from build123d import *

# Parameters (mm, degrees)
F0_W     = 20
F0_H     = 55
F1_DEPTH = 25.5
F3_DEPTH = 16
F5_DEPTH = 25
F7_D     = 5
F7_DEPTH = 10
F7_TIP   = 1.5021515476
F9_D     = 8
F9_DEPTH = 10
F9_TIP   = 2.4034424761


with BuildPart() as f1:
    # F0 (on Top) → F1 (new body)
    with BuildSketch(Plane.XY):
        Rectangle(F0_W, F0_H)
    extrude(amount=F1_DEPTH)

    # F2 (on face) → F3 (cut)
    with BuildSketch(Plane.XY.offset(25.5)):
        with BuildLine():
            Line((5, 10), (-5, 10))
            ThreePointArc((-5, 10), (-5.7071067812, 9.7071067812), (-6, 9))
            Line((-6, 9), (-6, -9))
            ThreePointArc((-6, -9), (-5.7071067812, -9.7071067812), (-5, -10))
            Line((-5, -10), (5, -10))
            ThreePointArc((5, -10), (5.7071067812, -9.7071067812), (6, -9))
            Line((6, -9), (6, 9))
            ThreePointArc((6, 9), (5.7071067812, 9.7071067812), (5, 10))
        make_face()
    extrude(amount=-F3_DEPTH, mode=Mode.SUBTRACT)

    # F4 (on face) → F5 (cut)
    with BuildSketch(Plane.YZ.offset(10)):
        Polygon((-27.5, 0), (-18, 0), (-15, 5.5), (-27.5, 5.5), align=None)
        Polygon((27.5, 5.5), (15, 5.5), (18, 0), (27.5, 0), align=None)
    extrude(amount=-F5_DEPTH, mode=Mode.SUBTRACT)

    # F7
    with Locations(Plane.YZ.offset(10)):
        with Locations((-17.5, 16.5), (17.5, 16.5)):
            Hole(F7_D / 2, depth=F7_DEPTH)
            with Locations((0, 0, -(F7_DEPTH + F7_TIP / 2))):  # 118° drill point
                Cone(0, F7_D / 2, F7_TIP, mode=Mode.SUBTRACT)

    # F9
    with Locations(Plane(origin=(-10, 0, 0), x_dir=(0, -1, 0), z_dir=(-1, 0, 0))):
        with Locations((0, 16.5)):
            Hole(F9_D / 2, depth=F9_DEPTH)
            with Locations((0, 0, -(F9_DEPTH + F9_TIP / 2))):  # 118° drill point
                Cone(0, F9_D / 2, F9_TIP, mode=Mode.SUBTRACT)


solid = f1.part
Here's how the part is built. I have some questions about the finished solid (model axes, mm). A direction names the side the tool comes from. Coordinates: 2 decimals unless noted, no trailing zeros. Order: outer loops, then holes, each group sorted by start corner. A loop starts at its lowest first (then second) coordinate and runs counter-clockwise, first axis right, second up. Notation, with made-up numbers: (-39, -24.5) - (3, -24.5) arc R25 ccw to (3, -1.5) - close; hole circle Ø2 at (18, 37.25). An arc over 180 degrees is marked (long way). Use CSV: the item, a comma, the result in double quotes. Start each with the question number.
1. Please list where these lines run through material, in increasing order: line 1 (X direction, y = 7.5, z = 22.5); line 2 (Y direction, x = 4.5, z = 20); line 3 (Y direction, x = 6.5, z = 16.5). Write a range as from..to.
2. Suppose I cut it at A-A on x = -8. List the corners of the cut face in (y, z) for me.
3. Suppose I cut it at C-C on x = -3.5. List the corners of the cut face in (y, z) for me.
4. If we mould it in two halves opening along Z, with no side actions, what happens to faces 4 (the face through (0, 0, 0)), 5 (the face through (-5.699, 9.715, 17.612)), 6 (the face through (4.9, -15, 16.6)), 7 (the face through (0.14, 16.48, 2.79))? For each: +Z half, -Z half, draft (parallel to the pull), parting line (faces both ways), or undercut.
5. Suppose I cut it at B-B on y = 0. List the corners of the cut face in (x, z) for me, then the cut area to 3 significant figures.
6. I'm going to push flat-ended pins straight in: pin 1 (10 mm diameter, centred on x = -2, y = 23.5, fed in from -Z); pin 2 (8 mm diameter, centred on y = -17.5, z = 16.5, fed in from +X); pin 3 (6 mm diameter, centred on x = -0.5, y = 5, fed in from +Z); pin 4 (1.5 mm diameter, centred on y = 0, z = 15, fed in from -X). Where does each tip first touch, or does it pass through?
7. Suppose I cut it at D-D on y = -6. List the corners of the cut face in (x, z) for me.
8. For faces 1 (the face through (6, 0, 18)), 2 (the face through (0.14, -16.52, 2.71)), 3 (the face through (4.9, 20, 16.6)), which set-ups out of +Z, -Z, +X, -X, +Y, -Y let a thin tool reach every point of the face, with its end or its side?
Output:
1,line 1,"x = -10..-6, 6..10"
1,line 2,"y = -27.5..-10, 10..27.5"
1,line 3,"y = -27.5..-20, -15..15, 20..27.5"
2,outline,"(-27.5, 5.5) - (-15, 5.5) - (-18, 0) - (18, 0) - (15, 5.5) - (27.5, 5.5) - (27.5, 25.5) - (-27.5, 25.5) - close; hole circle Ø8 at (0, 16.5)"
3,outline,"(-27.5, 5.5) - (-15, 5.5) - (-18, 0) - (18, 0) - (15, 5.5) - (27.5, 5.5) - (27.5, 25.5) - (10, 25.5) - (10, 9.5) - (-10, 9.5) - (-10, 25.5) - (-27.5, 25.5) - close"
4,face 4,"-Z half"
4,face 5,"draft"
4,face 6,"undercut"
4,face 7,"undercut"
5,outline,"(-10, 0) - (10, 0) - (10, 25.5) - (6, 25.5) - (6, 9.5) - (-6, 9.5) - (-6, 12.5) - (-10, 12.5) - close; (-10, 20.5) - (-6, 20.5) - (-6, 25.5) - (-10, 25.5) - close"
5,area,"286 mm2"
6,pin 1,"stops at z = 5.5"
6,pin 2,"stops at x = 10"
6,pin 3,"stops at z = 9.5"
6,pin 4,"stops at x = 6"
7,outline,"(-10, 0) - (10, 0) - (10, 25.5) - (6, 25.5) - (6, 9.5) - (-6, 9.5) - (-6, 25.5) - (-10, 25.5) - close"
8,face 1,"+Z"
8,face 2,"+X, -X, -Y"
8,face 3,"+X"
